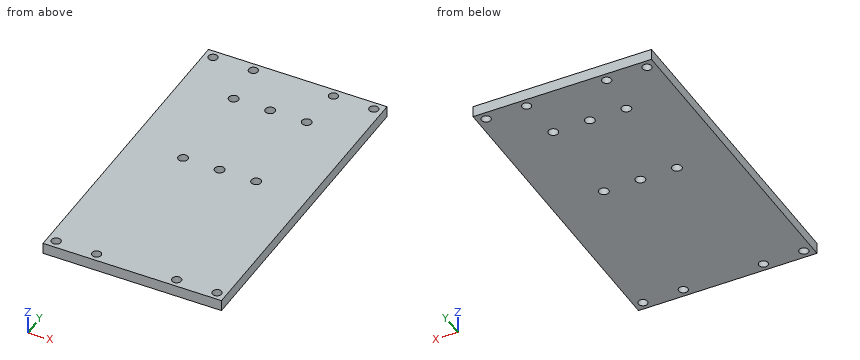
from build123d import *

# Parameters (mm, degrees)
ESBO_O1_W                = 101.6
ESBO_O1_H                = 180
RESSALTO_EXTRUS_O1_DEPTH = 6.35
CORTE_EXTRUS_O1_REACH    = 105.542
ESBO_O2_R                = 2.6
CORTE_EXTRUS_O2_REACH    = 105.542
ESBO_O3_R                = 2.75


with BuildPart() as part:
    # Esboço1 → Ressalto-extrusão1 (new body)
    with BuildSketch(Plane.XY):
        Rectangle(ESBO_O1_W, ESBO_O1_H)
    extrude(amount=RESSALTO_EXTRUS_O1_DEPTH)

    # Esboço2 → Corte-extrusão1 (cut, up to next)
    with BuildSketch(Plane.XY.offset(6.35), mode=Mode.PRIVATE) as corte_extrus_o1_sk1:
        with Locations((-45.8, 85.24)):
            Circle(ESBO_O2_R)
    corte_extrus_o1_tool1 = extrude(corte_extrus_o1_sk1.sketch, amount=-CORTE_EXTRUS_O1_REACH, mode=Mode.PRIVATE) & part.part
    # Esboço2 → Corte-extrusão1 (cut, up to next)
    with BuildSketch(Plane.XY.offset(6.35), mode=Mode.PRIVATE) as corte_extrus_o1_sk2:
        with Locations((-22.8, 85.24)):
            Circle(ESBO_O2_R)
    corte_extrus_o1_tool2 = extrude(corte_extrus_o1_sk2.sketch, amount=-CORTE_EXTRUS_O1_REACH, mode=Mode.PRIVATE) & part.part
    # Esboço2 → Corte-extrusão1 (cut, up to next)
    with BuildSketch(Plane.XY.offset(6.35), mode=Mode.PRIVATE) as corte_extrus_o1_sk3:
        with Locations((22.8, 85.24)):
            Circle(ESBO_O2_R)
    corte_extrus_o1_tool3 = extrude(corte_extrus_o1_sk3.sketch, amount=-CORTE_EXTRUS_O1_REACH, mode=Mode.PRIVATE) & part.part
    # Esboço2 → Corte-extrusão1 (cut, up to next)
    with BuildSketch(Plane.XY.offset(6.35), mode=Mode.PRIVATE) as corte_extrus_o1_sk4:
        with Locations((45.8, 85.24)):
            Circle(ESBO_O2_R)
    corte_extrus_o1_tool4 = extrude(corte_extrus_o1_sk4.sketch, amount=-CORTE_EXTRUS_O1_REACH, mode=Mode.PRIVATE) & part.part
    # Esboço2 → Corte-extrusão1 (cut, up to next)
    with BuildSketch(Plane.XY.offset(6.35), mode=Mode.PRIVATE) as corte_extrus_o1_sk5:
        with Locations((45.8, -85.24)):
            Circle(ESBO_O2_R)
    corte_extrus_o1_tool5 = extrude(corte_extrus_o1_sk5.sketch, amount=-CORTE_EXTRUS_O1_REACH, mode=Mode.PRIVATE) & part.part
    # Esboço2 → Corte-extrusão1 (cut, up to next)
    with BuildSketch(Plane.XY.offset(6.35), mode=Mode.PRIVATE) as corte_extrus_o1_sk6:
        with Locations((22.8, -85.24)):
            Circle(ESBO_O2_R)
    corte_extrus_o1_tool6 = extrude(corte_extrus_o1_sk6.sketch, amount=-CORTE_EXTRUS_O1_REACH, mode=Mode.PRIVATE) & part.part
    # Esboço2 → Corte-extrusão1 (cut, up to next)
    with BuildSketch(Plane.XY.offset(6.35), mode=Mode.PRIVATE) as corte_extrus_o1_sk7:
        with Locations((-22.8, -85.24)):
            Circle(ESBO_O2_R)
    corte_extrus_o1_tool7 = extrude(corte_extrus_o1_sk7.sketch, amount=-CORTE_EXTRUS_O1_REACH, mode=Mode.PRIVATE) & part.part
    # Esboço2 → Corte-extrusão1 (cut, up to next)
    with BuildSketch(Plane.XY.offset(6.35), mode=Mode.PRIVATE) as corte_extrus_o1_sk8:
        with Locations((-45.8, -85.24)):
            Circle(ESBO_O2_R)
    corte_extrus_o1_tool8 = extrude(corte_extrus_o1_sk8.sketch, amount=-CORTE_EXTRUS_O1_REACH, mode=Mode.PRIVATE) & part.part
    add(corte_extrus_o1_tool1.solids().sort_by_distance((-45.8, 85.24, 6.35))[0], mode=Mode.SUBTRACT)
    add(corte_extrus_o1_tool2.solids().sort_by_distance((-22.8, 85.24, 6.35))[0], mode=Mode.SUBTRACT)
    add(corte_extrus_o1_tool3.solids().sort_by_distance((22.8, 85.24, 6.35))[0], mode=Mode.SUBTRACT)
    add(corte_extrus_o1_tool4.solids().sort_by_distance((45.8, 85.24, 6.35))[0], mode=Mode.SUBTRACT)
    add(corte_extrus_o1_tool5.solids().sort_by_distance((45.8, -85.24, 6.35))[0], mode=Mode.SUBTRACT)
    add(corte_extrus_o1_tool6.solids().sort_by_distance((22.8, -85.24, 6.35))[0], mode=Mode.SUBTRACT)
    add(corte_extrus_o1_tool7.solids().sort_by_distance((-22.8, -85.24, 6.35))[0], mode=Mode.SUBTRACT)
    add(corte_extrus_o1_tool8.solids().sort_by_distance((-45.8, -85.24, 6.35))[0], mode=Mode.SUBTRACT)

    # Esboço3 → Corte-extrusão2 (cut, up to next)
    with BuildSketch(Plane.XY.offset(6.35), mode=Mode.PRIVATE) as corte_extrus_o2_sk1:
        with Locations((-20.8, 5)):
            Circle(ESBO_O3_R)
    corte_extrus_o2_tool1 = extrude(corte_extrus_o2_sk1.sketch, amount=-CORTE_EXTRUS_O2_REACH, mode=Mode.PRIVATE) & part.part
    # Esboço3 → Corte-extrusão2 (cut, up to next)
    with BuildSketch(Plane.XY.offset(6.35), mode=Mode.PRIVATE) as corte_extrus_o2_sk2:
        with Locations((0, 5)):
            Circle(ESBO_O3_R)
    corte_extrus_o2_tool2 = extrude(corte_extrus_o2_sk2.sketch, amount=-CORTE_EXTRUS_O2_REACH, mode=Mode.PRIVATE) & part.part
    # Esboço3 → Corte-extrusão2 (cut, up to next)
    with BuildSketch(Plane.XY.offset(6.35), mode=Mode.PRIVATE) as corte_extrus_o2_sk3:
        with Locations((20.8, 5)):
            Circle(ESBO_O3_R)
    corte_extrus_o2_tool3 = extrude(corte_extrus_o2_sk3.sketch, amount=-CORTE_EXTRUS_O2_REACH, mode=Mode.PRIVATE) & part.part
    # Esboço3 → Corte-extrusão2 (cut, up to next)
    with BuildSketch(Plane.XY.offset(6.35), mode=Mode.PRIVATE) as corte_extrus_o2_sk4:
        with Locations((20.8, 60)):
            Circle(ESBO_O3_R)
    corte_extrus_o2_tool4 = extrude(corte_extrus_o2_sk4.sketch, amount=-CORTE_EXTRUS_O2_REACH, mode=Mode.PRIVATE) & part.part
    # Esboço3 → Corte-extrusão2 (cut, up to next)
    with BuildSketch(Plane.XY.offset(6.35), mode=Mode.PRIVATE) as corte_extrus_o2_sk5:
        with Locations((0, 60)):
            Circle(ESBO_O3_R)
    corte_extrus_o2_tool5 = extrude(corte_extrus_o2_sk5.sketch, amount=-CORTE_EXTRUS_O2_REACH, mode=Mode.PRIVATE) & part.part
    # Esboço3 → Corte-extrusão2 (cut, up to next)
    with BuildSketch(Plane.XY.offset(6.35), mode=Mode.PRIVATE) as corte_extrus_o2_sk6:
        with Locations((-20.8, 60)):
            Circle(ESBO_O3_R)
    corte_extrus_o2_tool6 = extrude(corte_extrus_o2_sk6.sketch, amount=-CORTE_EXTRUS_O2_REACH, mode=Mode.PRIVATE) & part.part
    add(corte_extrus_o2_tool1.solids().sort_by_distance((-20.8, 5, 6.35))[0], mode=Mode.SUBTRACT)
    add(corte_extrus_o2_tool2.solids().sort_by_distance((0, 5, 6.35))[0], mode=Mode.SUBTRACT)
    add(corte_extrus_o2_tool3.solids().sort_by_distance((20.8, 5, 6.35))[0], mode=Mode.SUBTRACT)
    add(corte_extrus_o2_tool4.solids().sort_by_distance((20.8, 60, 6.35))[0], mode=Mode.SUBTRACT)
    add(corte_extrus_o2_tool5.solids().sort_by_distance((0, 60, 6.35))[0], mode=Mode.SUBTRACT)
    add(corte_extrus_o2_tool6.solids().sort_by_distance((-20.8, 60, 6.35))[0], mode=Mode.SUBTRACT)


solid = part.part
Geometry check sheet. Reference: the model listing, model coordinates, mm. Give positions to 0.01 mm unless a question says otherwise; leave off trailing zeros. Loops run counter-clockwise (first coordinate to the right, second up) from the corner with the lowest first, then second, coordinate; pieces in that order, holes last. Notation, with made-up numbers: M -11,68 L 43,68 A17 ccw 43,82 Z; hole C 17,51.5 d9. An arc over 180 degrees is marked long. Answer as a JSON object with one key per item and string values. Group by question number.
Item 1: Sectioned sample at D-D on y = -85.24. Record the boundary of the cut face in (x, z), plus the area to 3 significant figures.
Item 2: Sectioned sample at C-C on z = 4.75. Give the number of separate pieces and of enclosed holes in the cut face, plus the area to 3 significant figures.
Item 3: Material ranges on L1, parallel to Y at x = -45.8, z = 4.25; L2, parallel to Y at x = 0, z = 2.5; L3, parallel to Y at x = 20.8, z = 5, recorded low to high.
Item 4: Sectioned sample at B-B on y = 60. Record the boundary of the cut face in (x, z), plus the area to 3 significant figures.
Item 5: Sectioned sample at A-A on x = -45.8. Record the boundary of the cut face in (y, z).
Findings below:
{
 "1": {"outline": "M -50.8,0 L -48.4,0 L -48.4,6.35 L -50.8,6.35 Z; M -43.2,0 L -25.4,0 L -25.4,6.35 L -43.2,6.35 Z; M -20.2,0 L 20.2,0 L 20.2,6.35 L -20.2,6.35 Z; M 25.4,0 L 43.2,0 L 43.2,6.35 L 25.4,6.35 Z; M 48.4,0 L 50.8,0 L 50.8,6.35 L 48.4,6.35 Z", "area": "513 mm2"},
 "2": {"separate pieces": "1", "enclosed holes": "14", "area": "18,000 mm2"},
 "3": {"L1": "-90 to -87.84, -82.64 to 82.64, 87.84 to 90", "L2": "-90 to 2.25, 7.75 to 57.25, 62.75 to 90", "L3": "-90 to -86.9, -83.58 to 2.25, 7.75 to 57.25, 62.75 to 83.58, 86.9 to 90"},
 "4": {"outline": "M -50.8,0 L -23.55,0 L -23.55,6.35 L -50.8,6.35 Z; M -18.05,0 L -2.75,0 L -2.75,6.35 L -18.05,6.35 Z; M 2.75,0 L 18.05,0 L 18.05,6.35 L 2.75,6.35 Z; M 23.55,0 L 50.8,0 L 50.8,6.35 L 23.55,6.35 Z", "area": "540 mm2"},
 "5": {"outline": "M -90,0 L -87.84,0 L -87.84,6.35 L -90,6.35 Z; M -82.64,0 L 82.64,0 L 82.64,6.35 L -82.64,6.35 Z; M 87.84,0 L 90,0 L 90,6.35 L 87.84,6.35 Z"}
}
